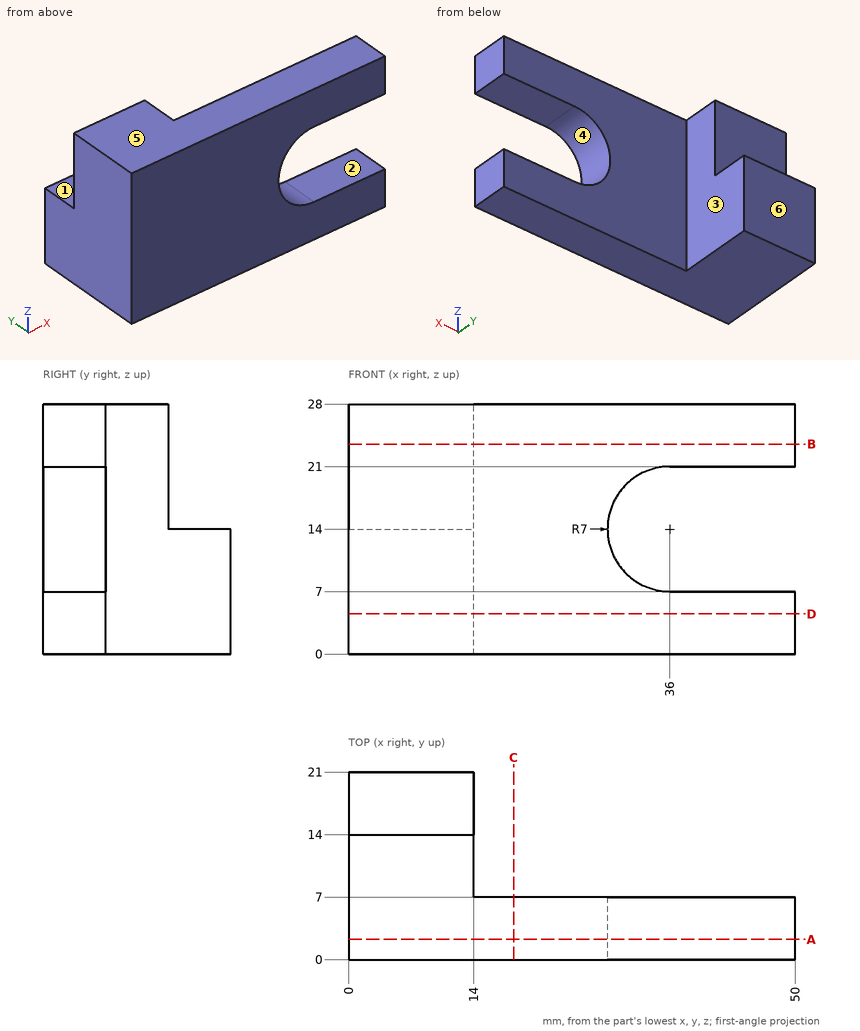
The drawing under review shows one solid part. Ordinate dimensions are in mm from its lowest x, y, z. A direction names the side the tool comes from. Coordinates: 2 decimals unless noted, no trailing zeros. Write each loop counter-clockwise with the first axis right and the second up, starting at its lowest first coordinate (ties: lowest second). Pieces come first, ordered by that corner, then holes. Notation, with made-up numbers: (0, 75.25) - (51, 75.25) arc R30 cw to (51, 110.25) - close; hole circle Ø1 at (2.5, -34). An arc over 180 degrees is marked (long way). Answer as CSV lines item,"result".
(1) Tool access review of the marked faces 1, 2 and 3: name each direction out of +Z, -Z, +X, -X, +Y, -Y from which nothing blocks a thin tool from reaching the whole face with its end or side.
Data:
face 1,"+Z, +X, -X, +Y"
face 2,"+X, +Y, -Y"
face 3,"+Z, -Z, +X, +Y"
(2) We need section A-A (y = 2.25). Give the boundary of the cut face in (x, z).
Data:
outline,"(0, 0) - (50, 0) - (50, 7) - (36, 7) arc R7 cw to (36, 21) - (50, 21) - (50, 28) - (0, 28) - close"
(3) We need section D-D (z = 4.5). Give the boundary of the cut face in (x, y).
Data:
outline,"(0, 0) - (50, 0) - (50, 7) - (14, 7) - (14, 21) - (0, 21) - close"
(4) Clearance check with flat-ended pins moving along their axes: pin 1 Ø12 at (x, z) = (28, 13) entering from -Y; pin 2 Ø15.5 at (x, z) = (10, 24.5) entering from +Y; pin 3 Ø2 at (x, y) = (4, 18) entering from +Z; pin 4 Ø10 at (x, z) = (34.5, 25) entering from +Y. State where each tip first meets the part, or that it passes through.
Data:
pin 1,"stops at y = 0"
pin 2,"stops at y = 14"
pin 3,"stops at z = 14"
pin 4,"stops at y = 7"
(5) We need section C-C (x = 18.5). Give the boundary of the cut face in (y, z).
Data:
outline,"(0, 0) - (7, 0) - (7, 28) - (0, 28) - close"
(6) Mouldability with a two-part tool opening along Z and no side actions: class the marked faces 4, 5 and 6 as pulls with the +Z half, pulls with the -Z half, needs draft (parallel to the pull), parting line crosses it, or undercut.
Data:
face 4,"undercut"
face 5,"pulls with the +Z half"
face 6,"needs draft"
(7) We need section B-B (z = 23.5). Give the boundary of the cut face in (x, y).
Data:
outline,"(0, 0) - (50, 0) - (50, 7) - (14, 7) - (14, 14) - (0, 14) - close"
(8) For line 1 along Z through (x, y) = (40, 4.25); line 2 along X through (y, z) = (13.25, 8); line 3 along Y through (x, z) = (40.5, 2), list the stretches that pass through material, from the lowest coordinate up. Write a range as [from, to].
Data:
line 1,"z = [0, 7], [21, 28]"
line 2,"x = [0, 14]"
line 3,"y = [0, 7]"
